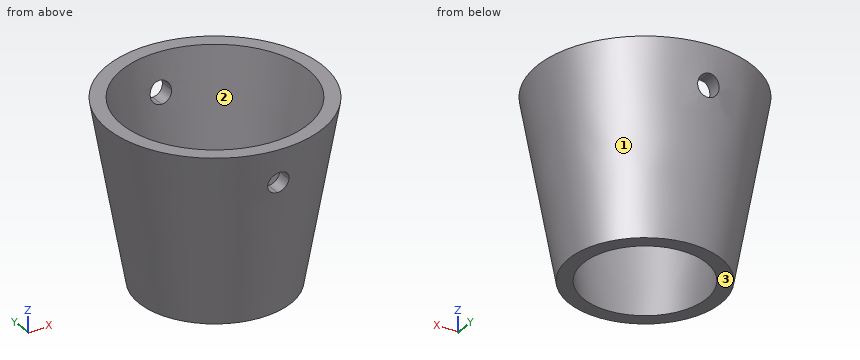
```python
from build123d import *

# Parameters (mm, degrees)
F3_DEPTH = 78.74


with BuildPart() as f1:
    # F0 (on Front) → F1 (revolve)
    with BuildSketch(Plane.XZ):
        with BuildLine():
            Line((0, 54.61), (0, 63.5))
            Line((0, 63.5), (-32.9416328116, 63.5))
            Line((-32.9416328116, 63.5), (-21.7448695366, 0))
            Line((-21.7448695366, 0), (0, 0))
            Line((0, 0), (0, 46.99))
            ThreePointArc((0, 46.99), (-3.81, 50.8), (0, 54.61))
        make_face()
        Polygon((-21.7448695366, 0), (-32.9416328116, 63.5), (-38.1, 63.5), (-26.903236725, 0), align=None)
    revolve(axis=Axis((0, 0, 31.75), (0, 0, 1)))

    # F0 (on Front) → F2 (revolve, cut)
    with BuildSketch(Plane.XZ):
        with BuildLine():
            Line((0, 54.61), (0, 63.5))
            Line((0, 63.5), (-32.9416328116, 63.5))
            Line((-32.9416328116, 63.5), (-21.7448695366, 0))
            Line((-21.7448695366, 0), (0, 0))
            Line((0, 0), (0, 46.99))
            ThreePointArc((0, 46.99), (-3.81, 50.8), (0, 54.61))
        make_face()
    revolve(axis=Axis((0, 0, 31.75), (0, 0, 1)), mode=Mode.SUBTRACT)

    # F0 (on Front) → F3 (cut, symmetric)
    with BuildSketch(Plane.XZ):
        with BuildLine():
            Line((0, 46.99), (0, 54.61))
            ThreePointArc((0, 54.61), (-3.81, 50.8), (0, 46.99))
        make_face()
        with BuildLine():
            ThreePointArc((3.81, 50.8), (2.6940768363, 53.4940768363), (0, 54.61))
            Line((0, 54.61), (0, 46.99))
            ThreePointArc((0, 46.99), (2.6940768363, 48.1059231637), (3.81, 50.8))
        make_face()
    extrude(amount=F3_DEPTH, both=True, mode=Mode.SUBTRACT)


solid = f1.part
```
Geometry check sheet. Reference: the model listing, model coordinates, mm. Face numbers are marked on the shaded views. Coordinates: 2 decimals unless noted, no trailing zeros. Order: outer loops, then holes, each group sorted by start corner. A loop starts at its lowest first (then second) coordinate and runs counter-clockwise, first axis right, second up. Notation, with made-up numbers: (21.25, -22) - (37.25, -22) arc R19 cw to (37.25, -11) - close; hole circle Ø11 at (76, -39.75). An arc over 180 degrees is marked (long way). Answer in a Markdown table with one row per item. Add a question column.
1. Section check C-C (z = 5). Enter the section's corners in (x, y).
2. Section check B-B (z = 35). Enter the section's corners in (x, y).
3. Gauge pin test, flat ends, axial feed: pin 1 Ø12 at (x, z) = (26.5, 46) entering from -Y; pin 2 Ø2 at (y, z) = (-2, 31.5) entering from -X; pin 3 Ø1 at (y, z) = (22.5, 45) entering from -X. Record the tip position at first contact, or that the pin passes through.
4. Section check A-A (y = 0). Enter the section's corners in (x, z).
5. Material ranges on L1, parallel to X at y = 3, z = 21.5; L2, parallel to Y at x = 23, z = 47.5; L3, parallel to Y at x = 18, z = 31.5, recorded low to high. Write a range as [from, to].
6. Draft check along X on the marked faces 1, 2 and 3. Enter one of: +X half, -X half, draft (parallel to the pull), parting line (faces both ways), or undercut.
Data:
| question | item | result |
|---|---|---|
| 1 | outline | circle Ø55.57 at (0, 0); hole circle Ø45.25 at (0, 0) |
| 2 | outline | circle Ø66.15 at (0, 0); hole circle Ø55.83 at (0, 0) |
| 3 | pin 1 | stops at y = -28.58 |
| 3 | pin 2 | stops at x = -32.58 |
| 3 | pin 3 | stops at x = -27.03 |
| 4 | outline | (-38.1, 63.5) - (-26.9, 0) - (-21.74, 0) - (-32.94, 63.5) - close; (21.74, 0) - (26.9, 0) - (38.1, 63.5) - (32.94, 63.5) - close |
| 5 | L1 | x = [-30.55, -25.36], [25.36, 30.55] |
| 5 | L2 | y = [-26.75, -19.45], [19.45, 26.75] |
| 5 | L3 | y = [-27.01, -20.52], [20.52, 27.01] |
| 6 | face 1 | parting line |
| 6 | face 2 | undercut |
| 6 | face 3 | draft |
